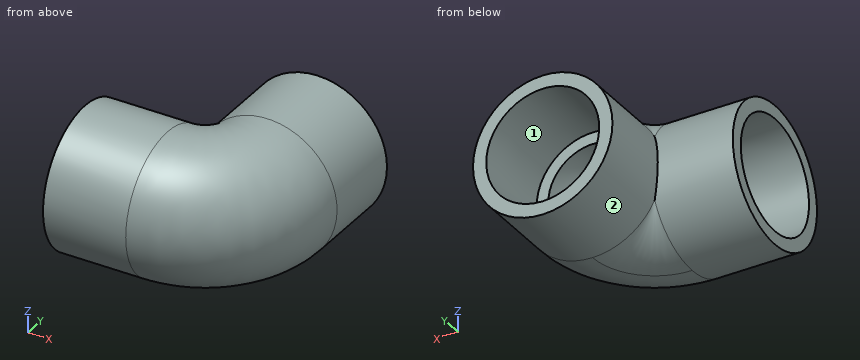
```python
from build123d import *

# Parameters (mm, degrees)
SKETCH3_R    = 29.972
SKETCH3_R_2  = 19.05
SCALE1_SCALE = 0.865


with BuildPart() as part:
    # Sketch1 → Revolve1 (revolve)
    with BuildSketch(Plane.XY, mode=Mode.PRIVATE) as revolve1_sk:
        Polygon((-62.23, -29.972), (-26.67, -29.972), (-26.67, -24.0538), (-62.23, -24.2824), align=None)
    revolve(revolve1_sk.sketch.rotate(Axis((-62.23, 0, 0), (1, 0, 0)), 270), axis=Axis((-62.23, 0, 0), (1, 0, 0)))


with BuildPart() as body_2:
    # Sketch2 → Revolve2 (revolve)
    with BuildSketch(Plane.XY, mode=Mode.PRIVATE) as revolve2_sk:
        Polygon((24.2824, 62.23), (24.0538, 26.67), (29.972, 26.67), (29.972, 62.23), align=None)
    revolve(revolve2_sk.sketch.rotate(Axis((0, 0, 0), (0, 1, 0)), 90), axis=Axis((0, 0, 0), (0, 1, 0)))


with BuildPart() as sweep1_tool:
    # Sweep1: sweep along a path in Sketch4
    with BuildLine(Plane.XY) as sweep1_path:
        ThreePointArc((-26.67, 0), (-7.811462, 7.811462), (0, 26.67))
    # Sketch3 → Sweep1 (sweep)
    with BuildSketch(Plane(origin=(-26.67, 0, 0), x_dir=(0, 0, -1), z_dir=(1, 0, 0))):
        Circle(SKETCH3_R)
        Circle(SKETCH3_R_2, mode=Mode.SUBTRACT)
    sweep(path=sweep1_path.line)


with BuildPart() as part_1:
    add(part.part)


with BuildPart() as part_2:
    # Sweep1: joined with sweep1_tool
    add(part_1.part.fuse(sweep1_tool.part, body_2.part, tol=0.00001))


with BuildPart() as part_3:
    # Scale1: scaled about (0, 0, 0)
    add(part_2.part.scale(SCALE1_SCALE))


solid = part_3.part
```
CAD build for the part. Positions are in the model's coordinates, mm. Face numbers are marked on the shaded views. Round coordinates to 2 decimals unless told otherwise and drop trailing zeros. Order: outer loops, then holes, each group sorted by start corner. A loop starts at its lowest first (then second) coordinate and runs counter-clockwise, first axis right, second up.
Item 1: Saw through at A-A on x = -34. Write the cut outline in (y, z), then the cut area to 3 significant figures.
Item 2: Saw through at B-B on y = 45. Write the cut outline in (x, z), then the cut area to 3 significant figures.
Item 3: Mould opens along Z. For the marked faces 1 and 2 say: pulls with the +Z half, pulls with the -Z half, needs draft (parallel to the pull), parting line crosses it, or undercut.
Item 4: Pin check, flat tips, straight feed: pin 1 (3 mm diameter, centred on y = -15, z = 9.5, fed in from +X); pin 2 (21 mm diameter, centred on y = 7.5, z = 6, fed in from -X); pin 3 (1.5 mm diameter, centred on y = -6.5, z = -8, fed in from -X). Stop position of each tip, or through.
Item 5: Probe line 1 along Z through (x, y) = (0, 20.5); line 2 along Y through (x, z) = (-18, -1.5); line 3 along Z through (x, y) = (13.5, 42). List the from-to ranges inside material, lowest first.
Reported:
1. outline: circle Ø51.85 at (0, 0); hole circle Ø41.75 at (0, 0)
1. area: 742 mm2
2. outline: circle Ø51.85 at (0, 0); hole circle Ø41.9 at (0, 0)
2. area: 733 mm2
3. face 1: undercut
3. face 2: parting line crosses it
4. pin 1: stops at x = 6.97
4. pin 2: stops at x = -23.07
4. pin 3: stops at x = -1.28
5. line 1: z = -25.93 to -16.48, 16.48 to 25.93
5. line 2: y = -25.62 to -16.08, 18.75 to 23.07
5. line 3: z = -22.13 to -15.99, 15.99 to 22.13
